Read the model definition and answer for the solid it produces. Units are mm, in the model's axes. A direction names the side the tool comes from. Round coordinates to 2 decimals unless told otherwise and drop trailing zeros. Order: outer loops, then holes, each group sorted by start corner. A loop starts at its lowest first (then second) coordinate and runs counter-clockwise, first axis right, second up. Notation, with made-up numbers: (10.25, 42) -> (34.25, 42) arc R16 ccw to (34.25, 50) -> close; hole circle Ø5 at (-10.75, 76). An arc over 180 degrees is marked (long way). Answer as a JSON object with one key per item and string values. Group by question number.
Item 1: The mould has two halves that part along Y. Classify faces 1 (the flat face through (3.3, -0.1, 0)), 2 (the cylindrical face through (-3, 0, -6)), 3 (the flat face through (1.267, -2.155, 4.521)): pulls with the +Y half, pulls with the -Y half, needs draft (parallel to the pull), parting line crosses it, or undercut.
Item 2: For faces 4 (the flat face through (1.233, 2.175, 4.521)), 5 (the flat face through (2, 2, 6)), determine the directions among +Z, -Z, +X, -X, +Y, -Y from which every point of the face is accessible in a straight line to the end or side of a thin tool.
Item 3: Consider probe 1 along Z at (x, y) = (0.5, 0.75); probe 2 along Y at (x, z) = (4, 1.75); probe 3 along Z at (x, y) = (-0.5, 4.25). Determine where each line is inside the solid, lowest interval first. Write a range as from..to.
Item 4: Section D-D, the plane z = -4 is taken. Write down the section's boundary in (x, y).
Item 5: Section B-B, the plane y = 0 is taken. Write down the section's boundary in (x, z).
Item 6: Section C-C, the plane z = 2 is taken. Write down the section's boundary in (x, y).
Item 7: Given P1, Ø2.5, axis at x = -0.5, y = 1, coming from the +Z side; P2, Ø1.5, axis at y = 1.5, z = -2.5, coming from the +X side; P3, Ø1.5, axis at x = 3.5, z = 1, coming from the +Y side, each flat-ended and moving along its own axis, determine where each tip first touches the part or whether it passes through.
Item 8: Section A-A, the plane z = 4 is taken. Write down the section's boundary in (x, y), plus the area to 3 significant figures.
Solid Edge part; units mm, degrees
sketch "Sketch1" plane through (0, 0, 0) normal (0, -1, 0) x (1, 0, 0)
  line L0 (0, 6) -> (4.4, 6)
  line L1 (4.4, 6) -> (5, 5.4)
  line L2 (5, 5.4) -> (5, 0)
  line L3 (5, 0) -> (3, 0)
  line L4 (3, 0) -> (3, -11)
  line L5 (3, -11) -> (2, -12)
  line L6 (2, -12) -> (0, -12)
  line L7 (0, -12) -> (0, 6)
  dimension "D1" = 3
  dimension "D2" = 4.4
revolve "RevolvedProtrusion1" add sketch "Sketch1" angle 360 about axis through (0, 0, 54) along (0, 0, -1)
sketch "Sketch2" plane through (0, 0, 6) normal (0, 0, 1) x (0, 1, 0)
  line L0 (-2.8868, 0) -> (-1.4434, 2.5)
  line L1 (-1.4434, 2.5) -> (1.4434, 2.5)
  line L2 (1.4434, 2.5) -> (2.8868, 0)
  line L3 (2.8868, 0) -> (1.4434, -2.5)
  line L4 (1.4434, -2.5) -> (-1.4434, -2.5)
  line L5 (-1.4434, -2.5) -> (-2.8868, 0)
extrude "Cutout1" cut sketch "Sketch2" against normal blind 3
cosmetic_thread "Thread1"
properties material "Steel"
Values found:
{
 "1": {"face 1": "needs draft", "face 2": "parting line crosses it", "face 3": "undercut"},
 "2": {"face 4": "+Z", "face 5": "+Z, +X, -X, +Y, -Y"},
 "3": {"probe 1": "-12..3", "probe 2": "-3..3", "probe 3": "0..6"},
 "4": {"outline": "circle Ø6 at (0, 0)"},
 "5": {"outline": "(-5, 0) -> (-3, 0) -> (-3, -11) -> (-2, -12) -> (2, -12) -> (3, -11) -> (3, 0) -> (5, 0) -> (5, 5.4) -> (4.4, 6) -> (2.5, 6) -> (2.5, 3) -> (-2.5, 3) -> (-2.5, 6) -> (-4.4, 6) -> (-5, 5.4) -> close"},
 "6": {"outline": "circle Ø10 at (0, 0)"},
 "7": {"P1": "z = 3", "P2": "x = 2.9", "P3": "y = 4.18"},
 "8": {"outline": "circle Ø10 at (0, 0); hole (-2.5, -1.44) -> (0, -2.89) -> (2.5, -1.44) -> (2.5, 1.44) -> (0, 2.89) -> (-2.5, 1.44) -> close", "area": "56.9 mm2"}
}
